The figure shows three views and two pictorial views of one solid part (mm, origin at its lowest corner). Answer the questions. Coordinates: 2 decimals unless noted, no trailing zeros. Loops run counter-clockwise (first coordinate to the right, second up) from the corner with the lowest first, then second, coordinate; pieces in that order, holes last. Notation, with made-up numbers: M 5,-11 L 39,-11 A29 cw 39,12 Z; hole C 1.25,-33.5 d2. An arc over 180 degrees is marked long. One line per item, written item: value. Start each with the question number.
1. The part is cut by section C-C (z = 91). Write down the section's boundary in (x, y).
2. The part is cut by section A-A (y = 1.2). Write down the section's boundary in (x, z).
3. Flat-ended cylindrical pins translate along their axes: pin 1 (1.6 mm diameter, centred on y = 2, z = 12.5, fed in from -X); pin 2 (1.6 mm diameter, centred on x = 1.5, y = 1, fed in from +Z); pin 3 (1 mm diameter, centred on y = 1, z = 104.5, fed in from -X). Find the tip coordinate at first contact, or state that the pin passes through.
4. The part is cut by section B-B (x = 16.5). Write down the section's boundary in (y, z).
5. Consider probe 1 along X at (y, z) = (2.85, 17.5). Determine where the line is inside the solid, lowest interval first.
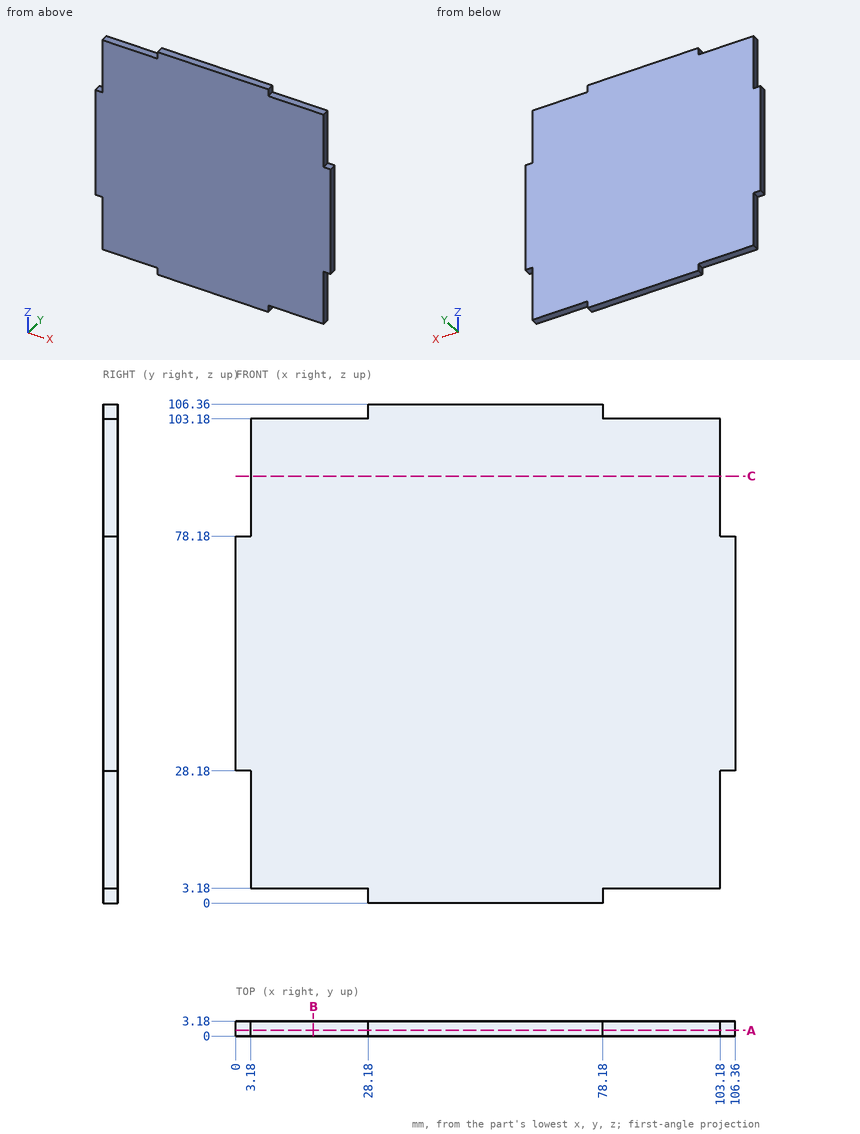
Answer block:
1. outline: M 3.18,0 L 103.18,0 L 103.18,3.18 L 3.18,3.18 Z
2. outline: M 0,28.18 L 3.18,28.18 L 3.18,3.18 L 28.18,3.18 L 28.18,0 L 78.18,0 L 78.18,3.18 L 103.18,3.18 L 103.18,28.18 L 106.36,28.18 L 106.36,78.18 L 103.18,78.18 L 103.18,103.18 L 78.18,103.18 L 78.18,106.36 L 28.18,106.36 L 28.18,103.18 L 3.18,103.18 L 3.18,78.18 L 0,78.18 Z
3. pin 1: stops at x = 3.18
3. pin 2: stops at z = 78.18
3. pin 3: stops at x = 28.18
4. outline: M 0,3.18 L 3.18,3.18 L 3.18,103.18 L 0,103.18 Z
5. probe 1: x = 3.18 to 103.18
